```python
from build123d import *

# Parameters (mm, degrees)
BOSS_EXTRUDE1_DEPTH = 12
CHAMFER1_SIZE       = 1


with BuildPart() as part:
    # Sketch1 → Boss-Extrude1 (new, symmetric)
    with BuildSketch(Plane.XY):
        Polygon((0, 0), (0, 40), (13, 40), (13, 10), (88, 10), (88, 6), (92, 6), (92, 10), (98, 10), (98, 0), align=None)
    extrude(amount=BOSS_EXTRUDE1_DEPTH, both=True)

    # Chamfer1
    chamfer1_edges = [part.edges().sort_by_distance(p)[0] for p in [
        (50.5, 10, -12),
        (95, 10, 12),
        (95, 10, -12),
        (50.5, 10, 12),
    ]]
    chamfer(chamfer1_edges, length=CHAMFER1_SIZE)


solid = part.part
```
Check sheet for the modelled part. Datum: model origin and axes. Units: mm. A direction names the side the tool comes from. Coordinates: 2 decimals unless noted, no trailing zeros. Write each loop counter-clockwise with the first axis right and the second up, starting at its lowest first coordinate (ties: lowest second). Pieces come first, ordered by that corner, then holes. Notation, with made-up numbers: (10.25, 37) - (37.25, 37) arc R22 ccw to (37.25, 68) - close; hole circle Ø3 at (28, 7.5). An arc over 180 degrees is marked (long way). One line per question, with ' | ' between items.
Item 1: Sectioned sample at A-A on x = 29.5. Record the boundary of the cut face in (y, z), plus the area to 3 significant figures.
Determined:
outline: (0, -12) - (9, -12) - (10, -11) - (10, 11) - (9, 12) - (0, 12) - close | area: 239 mm2
Item 2: Sectioned sample at B-B on z = -0.25. Record the boundary of the cut face in (x, y).
Determined:
outline: (0, 0) - (98, 0) - (98, 10) - (92, 10) - (92, 6) - (88, 6) - (88, 10) - (13, 10) - (13, 40) - (0, 40) - close
Item 3: Mould release check, pull along X, two halves, no side actions. Record for faces 4 (the face through (92, 8, 0)), 5 (the face through (31, 8, 12)), 6 (the face through (98, 5, 0)), 7 (the face through (90, 6, 0)): pulls with the +X half, pulls with the -X half, needs draft (parallel to the pull), parting line crosses it, or undercut.
Determined:
face 4: undercut | face 5: needs draft | face 6: pulls with the +X half | face 7: undercut
Item 4: Access from +Z, -Z, +X, -X, +Y, -Y to the whole of each face (thin tool, end or side, straight path). Record for faces 1 (the face through (50, 10, 0)), 2 (the face through (31, 8, -12)), 3 (the face through (88, 8, 0)).
Determined:
face 1: +Z, -Z, +X, +Y | face 2: -Z, +X, -X, +Y, -Y | face 3: +Z, -Z, +Y
Item 5: Thickness scan on line 1 (X direction, y = 8.5, z = -10); line 2 (X direction, y = 32, z = -5.5); line 3 (Y direction, x = 16.5, z = -6.75). Record the ranges inside material, lowest first. Write a range as [from, to].
Determined:
line 1: x = [0, 88], [92, 98] | line 2: x = [0, 13] | line 3: y = [0, 10]
Item 6: Sectioned sample at C-C on y = 26. Record the boundary of the cut face in (x, z).
Determined:
outline: (0, -12) - (13, -12) - (13, 12) - (0, 12) - close
Item 7: Gauge pin test, flat ends, axial feed: P1, Ø5, axis at x = 95, z = -1.5, coming from the +Y side; P2, Ø4, axis at y = 32, z = -8.5, coming from the -X side; P3, Ø6, axis at y = 21.5, z = 7, coming from the +X side; P4, Ø2, axis at x = 90, z = -6, coming from the +Y side. Record the tip position at first contact, or that the pin passes through.
Determined:
P1: stops at y = 10 | P2: stops at x = 0 | P3: stops at x = 13 | P4: stops at y = 6
